Verification items for the finished model (mm, model axes). Round coordinates to 2 decimals unless told otherwise and drop trailing zeros. Write each loop counter-clockwise with the first axis right and the second up, starting at its lowest first coordinate (ties: lowest second). Pieces come first, ordered by that corner, then holes. Notation, with made-up numbers: M 77,53 L 106,53 A17 cw 106,61 Z; hole C 47,89.5 d11. An arc over 180 degrees is marked long. Write each question's results on one line, items separated by ' | '.
Autodesk Inventor part; units mm, degrees
ref_plane "作業平面1" through (-29.5, 0, 0) normal (1, 0, 0) x (0, 0, -1)
ref_plane "YZ Plane" through (0, 0, 0) normal (1, 0, 0) x (0, 1, 0)
ref_plane "XZ Plane" through (0, 0, 0) normal (0, 1, 0) x (-1, 0, 0)
sketch "スケッチ1" plane through (0, 0, 0) normal (1, 0, 0) x (0, 1, 0)
  line L0 (0, 0) -> (6, 0)
  line L1 (6, 0) -> (6, -5)
  line L2 (6, -5) -> (0, -5)
  line L3 (0, -5) -> (0, 0)
  point P0 (3, -2.5)
  dimension "d0" = 6
  dimension "d1" = 5
  dimension "d2" = 3
  dimension "d3" = 2.5
extrude "押し出し1" add sketch "スケッチ1" against normal blind 27
ref_plane "作業平面1" through (-29.5, 0, 0) normal (1, 0, 0) x (0, 0, -1)
hole "穴1" at (0, 3, -2.5) direction (-1, 0, 0) diameter 2.5 end through all
sketch "スケッチ3" plane through (0, 0, -5) normal (0, 0, -1) x (-1, 0, 0)
  line L0 (0, 0) -> (27, 0)
  line L1 (0, 0) -> (0, 6)
  point P0 (13.5, 3)
  dimension "d19" = 3
  dimension "d20" = 13.5
hole "穴2" at (-13.5, 3, -5) direction (0, 0, 1) diameter 2.5 end through all
properties part number "belt_liner_v5_Plate_9" material "アルミニウム 6061"
1) Sectioned sample at A-A, the plane x = -14.25. Record the cut outline in (y, z).
Calculated:
outline: M 0,-5 L 2,-5 L 2,-3.25 A1.25 cw 2,-1.75 L 2,0 L 0,0 Z; M 4,-5 L 6,-5 L 6,0 L 4,0 L 4,-1.75 A1.25 cw 4,-3.25 Z
2) Draft check along X on faces 1 (the flat face through (0, 2, -1)), 2 (the cylindrical face through (-14.345, 2.079, -0.955)), 3 (the cylindrical face through (-12.74, 2.01, -4.01)), 4 (the flat face through (-27, 2, -1)). Enter one of: pulls with the +X half, pulls with the -X half, needs draft (parallel to the pull), parting line crosses it, or undercut.
Calculated:
face 1: pulls with the +X half | face 2: undercut | face 3: undercut | face 4: pulls with the -X half
3) Sectioned sample at D-D, the plane z = -3.2. Record the cut outline in (x, y).
Calculated:
outline: M -27,0 L 0,0 L 0,1.96 L -12.8,1.96 A1.25 cw -14.2,1.96 L -27,1.96 Z; M -27,4.04 L -14.2,4.04 A1.25 cw -12.8,4.04 L 0,4.04 L 0,6 L -27,6 Z
4) Sectioned sample at B-B, the plane y = 2.65. Record the cut outline in (x, z).
Calculated:
outline: M -27,-5 L -14.7,-5 L -14.7,-3.7 L -27,-3.7 Z; M -27,-1.3 L -14.7,-1.3 L -14.7,0 L -27,0 Z; M -12.3,-5 L 0,-5 L 0,-3.7 L -12.3,-3.7 Z; M -12.3,-1.3 L 0,-1.3 L 0,0 L -12.3,0 Z
5) Sectioned sample at C-C, the plane x = -8.5. Record the cut outline in (y, z), and give its area (3 significant figures).
Calculated:
outline: M 0,-5 L 6,-5 L 6,0 L 0,0 Z; hole C 3,-2.5 d2.5 | area: 25.1 mm²
6) Depth check by flat-ended pin: P1, Ø2, axis at x = -13.5, y = 3, coming from the +Z side. Enter the tip coordinate at first touch or a pass-through.
Calculated:
P1: passes through
7) Material ranges on line 1 (Z direction, x = -22.5, y = 3); line 2 (Y direction, x = -17.25, z = -2.5); line 3 (X direction, y = 3.1, z = -0.8), recorded low to high. Write a range as [from, to].
Calculated:
line 1: z = [-5, -3.75], [-1.25, 0] | line 2: y = [0, 1.75], [4.25, 6] | line 3: x = [-27, -14.75], [-12.25, 0]
